```python
from build123d import *

# Parameters (mm, degrees)
F3_R      = 0.85
F4_DEPTH  = 20
F2_R      = 4.5
F5_DEPTH  = 50
F6_START  = 4
F2_R_2    = 0.8
F6_DEPTH  = 21
F7_DEPTH  = 25
F8_START  = 6
F8_DEPTH  = 19
F9_START  = 6
F9_DEPTH  = 19
F13_SIZE  = 1
F14_START = -18.5
F14_DEPTH = 6.5
F15_START = -10
F15_DEPTH = 15


with BuildPart() as f4:
    # F3 (on Front) → F4 (new body)
    with BuildSketch(Plane.XZ):
        Polygon((14.9801738807, -12.5709681619), (14.9801738807, 19.1251428629), (-18.0198261193, 19.1251428629), (-18.0198261193, -16.8748571371), (10.6762849054, -16.8748571371), align=None)
        Polygon((-16.5198261193, 17.6251428629), (13.4801738807, 17.6251428629), (13.4801738807, -11.6982692705), (9.803586014, -15.3748571371), (-16.5198261193, -15.3748571371), align=None, mode=Mode.SUBTRACT)
        Polygon((13.4801738807, -11.6982692705), (13.4801738807, 17.6251428629), (-16.5198261193, 17.6251428629), (-16.5198261193, -15.3748571371), (9.803586014, -15.3748571371), align=None)
        with Locations((-14.5791273393, -13.3661682528)):
            Circle(F3_R, mode=Mode.SUBTRACT)
        with Locations((11.6150360554, 15.5776236206)):
            Circle(F3_R, mode=Mode.SUBTRACT)
        with Locations((11.6150360554, 15.5776236206)):
            Circle(F3_R)
        with Locations((-14.5791273393, -13.3661682528)):
            Circle(F3_R)
    extrude(amount=-F4_DEPTH)

    # F2 (on line) → F5 (cut)
    with BuildSketch(Plane(origin=(-1.2431124909, 4.6393589756, 0.846901634), x_dir=(-0.9669708455, -0.2507434208, -0.0457724901), z_dir=(-0.2548870022, 0.9512512426, 0.1736481777))):
        with Locations((0, 1.2139233295)):
            Circle(F2_R)
    extrude(amount=-F5_DEPTH, mode=Mode.SUBTRACT)

    # F2 (on line) → F6 (cut)
    with BuildSketch(Plane(origin=(-1.2431124909, 4.6393589756, 0.846901634), x_dir=(-0.9669708455, -0.2507434208, -0.0457724901), z_dir=(-0.2548870022, 0.9512512426, 0.1736481777)).offset(F6_START)):
        with BuildLine():
            Line((13.4, -14.7860766705), (13.4, 11.2139233295))
            Line((13.4, 11.2139233295), (8.9, 11.2139233295))
            Line((8.9, 11.2139233295), (7.5141987763, 11.2139233295))
            Line((7.5141987763, 11.2139233295), (7.5141987763, -1.0798760923))
            Line((7.5141987763, -1.0798760923), (10.4285785928, -2.7891881764))
            Line((10.4285785928, -2.7891881764), (10.4285785928, -10.4892711845))
            ThreePointArc((10.4285785928, -10.4892711845), (11.0398439007, -10.6956797169), (11.3, -11.2860766705))
            ThreePointArc((11.3, -11.2860766705), (11.0656854249, -11.8517620955), (10.5, -12.0860766705))
            Line((10.5, -12.0860766705), (0, -12.0860766705))
            Line((0, -12.0860766705), (-10.5, -12.0860766705))
            ThreePointArc((-10.5, -12.0860766705), (-11.2992009725, -11.250330264), (-10.4285785928, -10.4892711845))
            Line((-10.4285785928, -10.4892711845), (-10.4285785928, -2.7891881764))
            Line((-10.4285785928, -2.7891881764), (-7.5141987763, -1.0798760923))
            Line((-7.5141987763, -1.0798760923), (-7.5141987763, 11.2139233295))
            Line((-7.5141987763, 11.2139233295), (-8.9, 11.2139233295))
            Line((-8.9, 11.2139233295), (-13.4, 11.2139233295))
            Line((-13.4, 11.2139233295), (-13.4, -14.7860766705))
            Line((-13.4, -14.7860766705), (13.4, -14.7860766705))
        make_face()
        with Locations((-10.5, 1.2139233295)):
            Circle(F2_R_2, mode=Mode.SUBTRACT)
        with Locations((10.5, 1.2139233295)):
            Circle(F2_R_2, mode=Mode.SUBTRACT)
        with Locations((-10.5, 1.2139233295)):
            Circle(F2_R_2)
        with Locations((10.5, 1.2139233295)):
            Circle(F2_R_2)
        with BuildLine():
            ThreePointArc((-9.7, -11.2860766705), (-9.9096030464, -10.7462327698), (-10.4285785928, -10.4892711845))
            ThreePointArc((-10.4285785928, -10.4892711845), (-11.2992009725, -11.250330264), (-10.5, -12.0860766705))
            ThreePointArc((-10.5, -12.0860766705), (-9.9343145751, -11.8517620955), (-9.7, -11.2860766705))
        make_face()
        with BuildLine():
            ThreePointArc((11.3, -11.2860766705), (11.0398439007, -10.6956797169), (10.4285785928, -10.4892711845))
            ThreePointArc((10.4285785928, -10.4892711845), (9.7007990275, -11.321823077), (10.5, -12.0860766705))
            ThreePointArc((10.5, -12.0860766705), (11.0656854249, -11.8517620955), (11.3, -11.2860766705))
        make_face()
    extrude(amount=F6_DEPTH, mode=Mode.SUBTRACT)

    # F2 (on line) → F7 (cut)
    with BuildSketch(Plane(origin=(-1.2431124909, 4.6393589756, 0.846901634), x_dir=(-0.9669708455, -0.2507434208, -0.0457724901), z_dir=(-0.2548870022, 0.9512512426, 0.1736481777))):
        with BuildLine():
            Line((7.5141987763, -1.0798760923), (7.5141987763, 11.2139233295))
            Line((7.5141987763, 11.2139233295), (-7.5141987763, 11.2139233295))
            Line((-7.5141987763, 11.2139233295), (-7.5141987763, -1.0798760923))
            Line((-7.5141987763, -1.0798760923), (-10.4285785928, -2.7891881764))
            Line((-10.4285785928, -2.7891881764), (-10.4285785928, -10.4892711845))
            ThreePointArc((-10.4285785928, -10.4892711845), (-9.9096030464, -10.7462327698), (-9.7, -11.2860766705))
            ThreePointArc((-9.7, -11.2860766705), (-9.9343145751, -11.8517620955), (-10.5, -12.0860766705))
            Line((-10.5, -12.0860766705), (0, -12.0860766705))
            Line((0, -12.0860766705), (10.5, -12.0860766705))
            ThreePointArc((10.5, -12.0860766705), (9.7007990275, -11.321823077), (10.4285785928, -10.4892711845))
            Line((10.4285785928, -10.4892711845), (10.4285785928, -2.7891881764))
            Line((10.4285785928, -2.7891881764), (7.5141987763, -1.0798760923))
        make_face()
        with Locations((0, 1.2139233295)):
            Circle(F2_R, mode=Mode.SUBTRACT)
        with Locations((0, 1.2139233295)):
            Circle(F2_R)
        with Locations((10.5, 1.2139233295)):
            Circle(F2_R_2)
        with Locations((-10.5, 1.2139233295)):
            Circle(F2_R_2)
        with BuildLine():
            ThreePointArc((-9.7, -11.2860766705), (-9.9096030464, -10.7462327698), (-10.4285785928, -10.4892711845))
            ThreePointArc((-10.4285785928, -10.4892711845), (-11.2992009725, -11.250330264), (-10.5, -12.0860766705))
            ThreePointArc((-10.5, -12.0860766705), (-9.9343145751, -11.8517620955), (-9.7, -11.2860766705))
        make_face()
        with BuildLine():
            ThreePointArc((11.3, -11.2860766705), (11.0398439007, -10.6956797169), (10.4285785928, -10.4892711845))
            ThreePointArc((10.4285785928, -10.4892711845), (9.7007990275, -11.321823077), (10.5, -12.0860766705))
            ThreePointArc((10.5, -12.0860766705), (11.0656854249, -11.8517620955), (11.3, -11.2860766705))
        make_face()
    extrude(amount=F7_DEPTH, mode=Mode.SUBTRACT)

    # F2 (on line) → F8 (cut)
    with BuildSketch(Plane(origin=(-1.2431124909, 4.6393589756, 0.846901634), x_dir=(-0.9669708455, -0.2507434208, -0.0457724901), z_dir=(-0.2548870022, 0.9512512426, 0.1736481777)).offset(F8_START)):
        Polygon((7.5141987763, 11.2139233295), (8.9, 11.2139233295), (8.9, 13.3604565635), (-8.9, 13.3604565635), (-8.9, 11.2139233295), (-7.5141987763, 11.2139233295), align=None)
    extrude(amount=F8_DEPTH, mode=Mode.SUBTRACT)

    # F2 (on line) → F9 (cut)
    with BuildSketch(Plane(origin=(-1.2431124909, 4.6393589756, 0.846901634), x_dir=(-0.9669708455, -0.2507434208, -0.0457724901), z_dir=(-0.2548870022, 0.9512512426, 0.1736481777)).offset(F9_START)):
        Polygon((-8.9, 13.3604565635), (8.9, 13.3604565635), (8.8780205697, 15.9147679806), (-8.9, 15.9147679806), align=None)
    extrude(amount=F9_DEPTH, mode=Mode.SUBTRACT)

    # F11 (on line) → F12 (revolve, cut)
    with BuildSketch(Plane(origin=(0.0191665666, 0.0050521779, 0.0009222605), x_dir=(0.2543172943, -0.967043413, 0.0122372884), z_dir=(-0.9659258263, -0.2546115422, -0.0464786045))):
        Polygon((5.9364409902, 0.3417365793), (-3.8125691497, 2.0439563921), (-4.4443800577, -1.574572133), (2.9824459925, -14.1161987558), align=None)
    revolve(axis=Axis((0.3963748827, -1.6273101694, 1.1038607146), (0.2587939631, -0.9526311498, -0.1597484808)), mode=Mode.SUBTRACT)

    # F13
    f13_edges = [f4.edges().sort_by_distance(p)[0] for p in [
        (-3.671771, 0, -16.874857),
        (12.828229, 0, -14.722913),
        (14.980174, 0, 3.277087),
        (14.980174, 20, 3.277087),
        (12.828229, 20, -14.722913),
        (-3.671771, 20, -16.874857),
        (-18.019826, 10, 19.125143),
        (-18.019826, 10, -16.874857),
        (14.980174, 10, 19.125143),
        (-1.519826, 0, 19.125143),
        (-18.019826, 0, 1.125143),
        (9.046352, 20, 19.125143),
        (-16.649363, 20, 19.125143),
        (-18.019826, 20, -14.127167),
        (-18.019826, 20, 17.08766),
    ]]
    chamfer(f13_edges, length=F13_SIZE)

    # F3 (on Front) → F14 (cut)
    with BuildSketch(Plane.XZ.offset(F14_START)):
        Polygon((13.4801738807, -11.6982692705), (13.4801738807, 17.6251428629), (-16.5198261193, 17.6251428629), (-16.5198261193, -15.3748571371), (9.803586014, -15.3748571371), align=None)
        with Locations((-14.5791273393, -13.3661682528)):
            Circle(F3_R, mode=Mode.SUBTRACT)
        with Locations((11.6150360554, 15.5776236206)):
            Circle(F3_R, mode=Mode.SUBTRACT)
    extrude(amount=-F14_DEPTH, mode=Mode.SUBTRACT)

    # F3 (on Front) → F15 (cut)
    with BuildSketch(Plane.XZ.offset(F15_START)):
        with Locations((11.6150360554, 15.5776236206)):
            Circle(F3_R)
        with Locations((-14.5791273393, -13.3661682528)):
            Circle(F3_R)
    extrude(amount=-F15_DEPTH, mode=Mode.SUBTRACT)


solid = f4.part
```
Here's how the part is built. I have some questions about the finished solid (model axes, mm). A direction names the side the tool comes from. Round coordinates to 2 decimals unless told otherwise and drop trailing zeros. Order: outer loops, then holes, each group sorted by start corner. A loop starts at its lowest first (then second) coordinate and runs counter-clockwise, first axis right, second up. Notation, with made-up numbers: M 18,28 L 42,28 A9 cw 42,40 Z; hole C 11.25,66 d1. An arc over 180 degrees is marked long. Answer as CSV lines item,"result".
Item 1: Please list where these lines run through material, in increasing order: L1, parallel to X at y = 11.5, z = 4; L2, parallel to Y at x = -14, z = -14.5; L3, parallel to Y at x = -13, z = -7. Write a range as [from, to].
From the geometry:
L1,"[-18.02, -17.03], [10.69, 14.98]"
L2,"[0, 18.5]"
L3,"[0, 7.13]"
Item 2: We'd pull the mould along Y, two halves only. Please class faces 1 (the flat face through (-16.52, 19, 16)), 2 (the flat face through (14.296, 0.698, 18.507)), 3 (the cylindrical face through (-12.64, 3.43, 2.1)): +Y half, -Y half, draft (parallel to the pull), parting line (faces both ways), or undercut.
From the geometry:
face 1,"draft"
face 2,"-Y half"
face 3,"undercut"
Item 3: Which directions (+Z, -Z, +X, -X, +Y, -Y) give clear straight access to the entire face, cutting with the end or side of a thin tool? Please do faces 4 (the flat face through (-16.52, 19, -13)), 5 (the flat face through (-17.53, 19.49, -13.6)).
From the geometry:
face 4,"+Y"
face 5,"+Z, -Z, -X, +Y"
Item 4: For pin 1 (4 mm diameter, centred on x = 5, z = 1, fed in from -Y); pin 2 (0.8 mm diameter, centred on y = 19.5, z = 16, fed in from +X); pin 3 (2 mm diameter, centred on x = -1.5, z = -4, fed in from -Y), each with a flat end and sliding along its axis, tell me the tip position at first contact or that it passes through.
From the geometry:
pin 1,"y = 2.58"
pin 2,"x = 14.88"
pin 3,"y = 1.88"
Item 5: Imagine slicing it at B-B on y = 12. Give the number of separate pieces and of enclosed holes in the cut face, and give its area (3 significant figures).
From the geometry:
separate pieces,"1"
enclosed holes,"2"
area,"404 mm2"
Item 6: Imagine slicing it at A-A on x = -9. List the corners of the cut face in (y, z) for me.
From the geometry:
outline,"M 0,-15.87 L 1,-16.87 L 19,-16.87 L 20,-15.87 L 20,-15.37 L 18.5,-15.37 L 18.5,-11.65 L 9.35,-13.32 L 8.87,-10.67 L 4.8,-11.41 L 2.88,-0.88 L 4.78,-0.22 L 2.57,11.87 L 6.72,12.63 L 5.87,17.25 L 16.15,19.13 L 1,19.13 L 0,18.13 Z"
